Build history of the part. All positions in model axes, mm. A direction names the side the tool comes from. Coordinates: 2 decimals unless noted, no trailing zeros. Loops run counter-clockwise (first coordinate to the right, second up) from the corner with the lowest first, then second, coordinate; pieces in that order, holes last. Notation, with made-up numbers: M -11,55 L 48,55 A23 cw 48,63 Z; hole C 80,69 d8. An arc over 180 degrees is marked long. Write each question's results on one line, items separated by ' | '. Start each with the question number.
from build123d import *

# Parameters (mm, degrees)
SKETCH1_R           = 10.795
BOSS_EXTRUDE1_DEPTH = 25.4
SKETCH2_R           = 10.795
SKETCH2_R_2         = 6.35
CUT_EXTRUDE1_DEPTH  = 9.525
FILLET3_R           = 0.635


with BuildPart() as part:
    # Sketch1 → Boss-Extrude1 (new body)
    with BuildSketch(Plane.XY):
        Circle(SKETCH1_R)
        with BuildLine():
            Line((1.5, -2), (1.5, 2))
            ThreePointArc((1.5, 2), (0, 2.5), (-1.5, 2))
            Line((-1.5, 2), (-1.5, -2))
            ThreePointArc((-1.5, -2), (0, -2.5), (1.5, -2))
        make_face(mode=Mode.SUBTRACT)
    extrude(amount=BOSS_EXTRUDE1_DEPTH)

    # Sketch2 → Cut-Extrude1 (cut, symmetric)
    with BuildSketch(Plane.XY.offset(12.7)):
        Circle(SKETCH2_R)
        Circle(SKETCH2_R_2, mode=Mode.SUBTRACT)
    extrude(amount=CUT_EXTRUDE1_DEPTH, both=True, mode=Mode.SUBTRACT)

    # Fillet3
    fillet3_edges = [part.edges().sort_by_distance(p)[0] for p in [
        (-10.795, 0, 0),
        (-10.795, 0, 3.175),
        (-10.795, 0, 22.225),
        (-10.795, 0, 25.4),
    ]]
    fillet(fillet3_edges, radius=FILLET3_R)


solid = part.part
1. Band-saw the part on B-B, the plane x = 0. List the corners of the cut face in (y, z) (3 decimals).
2. Band-saw the part on C-C, the plane z = 16. List the corners of the cut face in (x, y).
3. Mould opens along Z. For faces 1 (the flat face through (0, -7, 3.175)), 2 (the cylindrical face through (0, -2.5, 12.5)), 3 (the flat face through (2, 0, 25.4)) say: +Z half, -Z half, draft (parallel to the pull), parting line (faces both ways), or undercut.
4. Wall check: line 1 along Z through (x, y) = (-3.75, 5.5) (3 decimals); line 2 along Y through (x, z) = (0, 8.5); line 3 along X through (y, z) = (1.25, 5). Give the ranges that are in metal, low to high.
5. Which spindle directions (+Z, -Z, +X, -X, +Y, -Y) get a long thin tool onto all of the face, cutting with end or side? Do faces 4 (the flat face through (0, -7, 22.225)), 5 (the flat face through (2, 0, 0)), 6 (the cylindrical face through (0, 2.5, 12.5)). Say none if no direction does.
6. Band-saw the part on A-A, the plane y = 0. List the corners of the cut face in (x, z) (3 decimals), plus the area to 3 significant figures.
7. Pin check, flat tips, straight feed: pin 1 (6 mm diameter, centred on x = 5, z = 22, fed in from -Y); pin 2 (1.2 mm diameter, centred on y = -0.5, z = 15, fed in from -X); pin 3 (3 mm diameter, centred on y = 0.5, z = 7, fed in from +X). Stop position of each tip, or through.
Checked values:
1) outline: M -10.795,0.635 A0.635 ccw -10.16,0 L -2.5,0 L -2.5,25.4 L -10.16,25.4 A0.635 ccw -10.795,24.765 L -10.795,22.86 A0.635 ccw -10.16,22.225 L -6.35,22.225 L -6.35,3.175 L -10.16,3.175 A0.635 ccw -10.795,2.54 Z; M 2.5,0 L 10.16,0 A0.635 ccw 10.795,0.635 L 10.795,2.54 A0.635 ccw 10.16,3.175 L 6.35,3.175 L 6.35,22.225 L 10.16,22.225 A0.635 ccw 10.795,22.86 L 10.795,24.765 A0.635 ccw 10.16,25.4 L 2.5,25.4 Z
2) outline: C 0,0 d12.7; hole M -1.5,-2 A2.5 ccw 1.5,-2 L 1.5,2 A2.5 ccw -1.5,2 Z
3) face 1: undercut | face 2: draft | face 3: +Z half
4) line 1: 0 to 3.175, 22.225 to 25.4 | line 2: -6.35 to -2.5, 2.5 to 6.35 | line 3: -6.23 to -1.5, 1.5 to 6.23
5) face 4: none | face 5: -Z, +X, -X, +Y, -Y | face 6: +Z, -Z
6) outline: M -10.795,0.635 A0.635 ccw -10.16,0 L -1.5,0 L -1.5,25.4 L -10.16,25.4 A0.635 ccw -10.795,24.765 L -10.795,22.86 A0.635 ccw -10.16,22.225 L -6.35,22.225 L -6.35,3.175 L -10.16,3.175 A0.635 ccw -10.795,2.54 Z; M 1.5,0 L 10.16,0 A0.635 ccw 10.795,0.635 L 10.795,2.54 A0.635 ccw 10.16,3.175 L 6.35,3.175 L 6.35,22.225 L 10.16,22.225 A0.635 ccw 10.795,22.86 L 10.795,24.765 A0.635 ccw 10.16,25.4 L 1.5,25.4 Z | area: 302 mm²
7) pin 1: y = -10.58 | pin 2: x = -6.35 | pin 3: x = 6.35
